Source: CAD feature listing. Evaluate the final solid. Frame: model axes, mm. Give positions to 0.01 mm unless a question says otherwise; leave off trailing zeros. Order: outer loops, then holes, each group sorted by start corner. A loop starts at its lowest first (then second) coordinate and runs counter-clockwise, first axis right, second up. Notation, with made-up numbers: M 28,59.25 L 60,59.25 A28 ccw 60,95.25 Z; hole C 89,-25 d10. An arc over 180 degrees is marked long. Answer as a JSON object with one key per item and string values. Group by question number.
1. Section query A-A (y = 2.75). Count the separate pieces of the cut face and the enclosed holes in it, plus the area to 3 significant figures.
2. Section query B-B (z = 44). Output: boundary loops of the cut face in (x, y), plus the area to 3 significant figures.
3. Pin query (flat end, axial travel): P1, Ø4.5, axis at x = 107.09, z = -19.11, coming from the -Y side; P2, Ø3, axis at x = 63, y = 2, coming from the +Z side; P3, Ø2.5, axis at x = 19.05, z = -107.15, coming from the +Y side; P4, Ø1, axis at y = 5.5, z = -59, coming from the +X side. Return the tip coordinate at first contact, or that it passes through.
4. Section query C-C (x = 64). Output: boundary loops of the cut face in (y, z), plus the area to 3 significant figures.
5. Material intervals for L1, parallel to X at y = 4.25, z = -106; L2, parallel to Z at x = -106, y = 3; L3, parallel to Z at x = -19, y = 0.75, sorted ascending. Write a range as [from, to].
from build123d import *

# Parameters (mm, degrees)
SKETCH1_R           = 122.4
BOSS_EXTRUDE1_DEPTH = 6.35
SKETCH2_R           = 1.9939
CUT_EXTRUDE1_DEPTH  = 174.216172744
CIRPATTERN1_COUNT   = 4


with BuildPart() as part:
    # Sketch1 → Boss-Extrude1 (new body)
    with BuildSketch(Plane(origin=(0, 0, 0), x_dir=(1, 0, 0), z_dir=(0, 1, 0))):
        with Locations(Location((0, 0, 0), (0, 0, 270))):
            Circle(SKETCH1_R)
    extrude(amount=BOSS_EXTRUDE1_DEPTH)

    # Sketch2 → Cut-Extrude1 (cut, through all)
    with BuildSketch(Plane(origin=(0, 6.35, 0), x_dir=(1, 0, 0), z_dir=(0, 1, 0))):
        with Locations(Location((-19.05, -107.035541925, 0), (0, 0, 270))):
            Circle(SKETCH2_R)
        with Locations(Location((19.05, -107.035541925, 0), (0, 0, 270))):
            Circle(SKETCH2_R)
    cut_extrude1 = extrude(amount=-CUT_EXTRUDE1_DEPTH, mode=Mode.SUBTRACT)

    # CirPattern1: Cut-Extrude1 ×4 about axis
    cirpattern1_axis = Axis((0, 0, -0.056837174), (0, 1, 0))
    for i in range(1, CIRPATTERN1_COUNT):
        add(cut_extrude1.rotate(cirpattern1_axis, i * 360 / CIRPATTERN1_COUNT), mode=Mode.SUBTRACT)


solid = part.part
Answer sheet:
{
 "1": {"separate pieces": "1", "enclosed holes": "8", "area": "47,000 mm^2"},
 "2": {"outline": "M -114.22,0 L 114.22,0 L 114.22,6.35 L -114.22,6.35 Z", "area": "1,450 mm^2"},
 "3": {"P1": "y = 0", "P2": "z = 105.83", "P3": "through", "P4": "x = 107.52"},
 "4": {"outline": "M 0,-104.33 L 6.35,-104.33 L 6.35,104.33 L 0,104.33 Z", "area": "1,330 mm^2"},
 "5": {"L1": "[-61.2, -20.68], [-17.42, 17.42], [20.68, 61.2]", "L2": "[-61.2, -20.77], [-17.44, 17.33], [20.66, 61.2]", "L3": "[-120.92, -109.14], [-105.16, 105.04], [109.03, 120.92]"}
}
